Could you check a few things on this model? Use its own coordinates, in mm. Face numbers are marked on the shaded views. A direction names the side the tool comes from. Give positions to 0.01 mm unless a question says otherwise; leave off trailing zeros. Order: outer loops, then holes, each group sorted by start corner. A loop starts at its lowest first (then second) coordinate and runs counter-clockwise, first axis right, second up. Notation, with made-up numbers: (31.25, 52) -> (78.25, 52) arc R33 cw to (78.25, 84) -> close; hole circle Ø4 at (17, 7). An arc over 180 degrees is marked (long way). Write each question's results on one line, items separated by ' | '.
```python
from build123d import *

# Parameters (mm, degrees)
Y_KSEKLIK_EKSTR_ZYON2_DEPTH = 15


with BuildPart() as part:
    # Çizim3 → Yükseklik-Ekstrüzyon2 (new body)
    with BuildSketch(Plane.XY):
        with BuildLine():
            Line((0, 45), (22.5, 45))
            ThreePointArc((22.5, 45), (25, 42.5), (22.5, 40))
            Line((22.5, 40), (0, 40))
            ThreePointArc((0, 40), (-20, 20), (0, 0))
            ThreePointArc((0, 0), (25, -25), (0, -50))
            Line((0, -50), (-22.5, -50))
            ThreePointArc((-22.5, -50), (-25, -47.5), (-22.5, -45))
            Line((-22.5, -45), (0, -45))
            ThreePointArc((0, -45), (20, -25), (0, -5))
            ThreePointArc((0, -5), (-25, 20), (0, 45))
        make_face()
    extrude(amount=Y_KSEKLIK_EKSTR_ZYON2_DEPTH)


solid = part.part
```
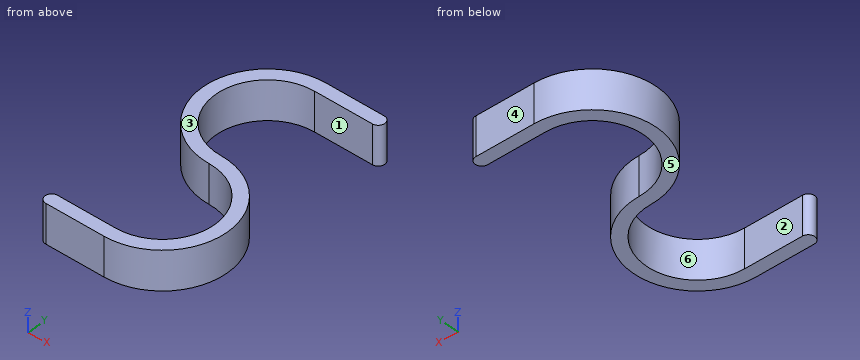
Q1. For the marked faces 1, 2 and 3, which set-ups out of +Z, -Z, +X, -X, +Y, -Y let a thin tool reach every point of the face, with its end or its side?
Here are the results:
face 1: +Z, -Z, +X | face 2: +Z, -Z, -X | face 3: +Z, +X, -X, +Y, -Y
Q2. I'm going to push flat-ended pins straight in: pin 1 Ø2 at (x, z) = (-18.5, 4.5) entering from +Y; pin 2 Ø4 at (y, z) = (20.5, 11.5) entering from +X; pin 3 Ø8 at (x, z) = (-10.5, 6) entering from +Y. Where does each tip first touch, or does it pass through?
Here are the results:
pin 1: stops at y = 37.85 | pin 2: stops at x = -19.84 | pin 3: stops at y = 44.14
Q3. Suppose I cut it at A-A on x = 5.5. Please give me the cut outline in (y, z), and give its area (3 significant figures).
Here are the results:
outline: (-49.39, 0) -> (-44.23, 0) -> (-44.23, 15) -> (-49.39, 15) -> close; (-5.77, 0) -> (-0.61, 0) -> (-0.61, 15) -> (-5.77, 15) -> close; (40, 0) -> (45, 0) -> (45, 15) -> (40, 15) -> close | area: 230 mm²
Q4. Thinking about a two-plate mould opening in Y: for the marked faces 4, 5 and 6, which applies, +Y half, -Y half, draft (parallel to the pull), parting line (faces both ways), or undercut?
Here are the results:
face 4: +Y half | face 5: draft | face 6: undercut
Q5. Suppose I cut it at D-D on x = -19. Please give me the cut outline in (y, z) (3 decimals).
Here are the results:
outline: (-50, 0) -> (-45, 0) -> (-45, 15) -> (-50, 15) -> close; (3.752, 0) -> (13.755, 0) -> (13.755, 15) -> (3.752, 15) -> close; (26.245, 0) -> (36.248, 0) -> (36.248, 15) -> (26.245, 15) -> close
Q6. Suppose I cut it at C-C on y = -25. Please give me the cut outline in (x, z), and give its area (3 significant figures).
Here are the results:
outline: (20, 0) -> (25, 0) -> (25, 15) -> (20, 15) -> close | area: 75.0 mm²
Q7. Suppose I cut it at B-B on z = 10. Please give me the cut outline in (x, y), and give its area (3 significant figures).
Here are the results:
outline: (-22.5, -50) -> (0, -50) arc R25 ccw to (0, 0) arc R20 cw to (0, 40) -> (22.5, 40) arc R2.5 ccw to (22.5, 45) -> (0, 45) arc R25 ccw to (0, -5) arc R20 cw to (0, -45) -> (-22.5, -45) arc R2.5 ccw to start | area: 951 mm²
Q8. I need wall thicknesses on line 1 along Y through (x, z) = (0.5, 8.5) (3 decimals); line 2 along Y through (x, z) = (-16.5, 9.25); line 3 along Y through (x, z) = (21.5, 3). Which ranges of each line are inside material? Lowest first, please.
Here are the results:
line 1: y = -49.995 to -44.994, -5.006 to -0.005, 40 to 45 | line 2: y = -50 to -45, 1.22 to 8.7, 31.3 to 38.78 | line 3: y = -37.76 to -12.24, 40 to 45
